For this review, take the finished solid that the model builds, in its own axes (mm). A direction names the side the tool comes from. Give positions to 0.01 mm unless a question says otherwise; leave off trailing zeros. Loops run counter-clockwise (first coordinate to the right, second up) from the corner with the lowest first, then second, coordinate; pieces in that order, holes last. Notation, with made-up numbers: (-7, 49) - (28, 49) arc R26 cw to (28, 78) - close; hole circle Ø2 at (-33, 49.25). An arc over 180 degrees is marked (long way). Put each result on its own line as item: value. Start each with the question number.
from build123d import *

# Parameters (mm, degrees)
SKETCH_1_W      = 10
SKETCH_1_H      = 12
EXTRUDE_1_DEPTH = 12
EXTRUDE_START   = 12
SKETCH_1_3_W    = 14
SKETCH_1_3_H    = 14
SKETCH_1_3_W_2  = 10
SKETCH_1_3_H_2  = 12
EXTRUDE_2_DEPTH = 3


with BuildPart() as part:
    # Эскиз1 → Бобышка-Вытянуть1 (new body)
    with BuildSketch(Plane(origin=(0, 0, 0), x_dir=(1, 0, 0), z_dir=(0, 1, 0))):
        Rectangle(SKETCH_1_W, SKETCH_1_H)
    extrude(amount=EXTRUDE_1_DEPTH)

    # Эскиз1<3> → Бобышка-Вытянуть2 (add)
    with BuildSketch(Plane(origin=(0, 0, 0), x_dir=(1, 0, 0), z_dir=(0, 1, 0)).offset(EXTRUDE_START)):
        Rectangle(SKETCH_1_3_W, SKETCH_1_3_H)
        Rectangle(SKETCH_1_3_W_2, SKETCH_1_3_H_2, mode=Mode.SUBTRACT)
        Rectangle(SKETCH_1_3_W_2, SKETCH_1_3_H_2)
    extrude(amount=EXTRUDE_2_DEPTH)


solid = part.part
1) Wall thickness on probe 1 along X at (y, z) = (1.5, -2.25); probe 2 along Z at (x, y) = (0.5, 6.5); probe 3 along Y at (x, z) = (-5.25, -5.75): over which ranges is each line inside the solid? List them lowest first.
2) Take a section at B-B on z = 0.25. State the section outline as (x, y) points.
3) Take a section at A-A on x = -4.5. State the section outline as (y, z) points.
4) Insertion check: P1, Ø8, axis at x = -0.5, y = 3.5, coming from the -Z side; P2, Ø6, axis at y = 4.5, z = -1.5, coming from the -X side; P3, Ø4, axis at y = 9.5, z = -4, coming from the +X side. Each pin has a flat end and moves straight along its axis. Give the tip position at first contact, or say it passes through.
5) Machinability: for faces 1 (the flat face through (0, 6, -6)), 2 (the flat face through (0, 6, 6)), 3 (the flat face through (5, 6, 0)), 4 (the flat face through (-5, 6, 0)), which of the approach directions +Z, -Z, +X, -X, +Y, -Y give a long, thin tool a straight path to every point of the face, cutting with its end or side? Answer none if there is none.
6) Take a section at D-D on x = -6. State the section outline as (y, z) points.
7) Take a section at C-C on y = 4. State the section outline as (x, z) points.
Answers follow:
1. probe 1: -5 to 5
1. probe 2: -6 to 6
1. probe 3: 12 to 15
2. outline: (-7, 12) - (-5, 12) - (-5, 0) - (5, 0) - (5, 12) - (7, 12) - (7, 15) - (-7, 15) - close
3. outline: (0, -6) - (12, -6) - (12, -7) - (15, -7) - (15, 7) - (12, 7) - (12, 6) - (0, 6) - close
4. P1: z = -6
4. P2: x = -5
4. P3: x = 5
5. face 1: -Z, +X, -X, -Y
5. face 2: +Z, +X, -X, -Y
5. face 3: +Z, -Z, +X, -Y
5. face 4: +Z, -Z, -X, -Y
6. outline: (12, -7) - (15, -7) - (15, 7) - (12, 7) - close
7. outline: (-5, -6) - (5, -6) - (5, 6) - (-5, 6) - close
